```python
from build123d import *

# Parameters (mm, degrees)
EXTRUDE_1_DEPTH          = 30
CUT_EXTRUDE_1_DEPTH      = 301
CUT_EXTRUDE_2_DEPTH      = 12
CUT_EXTRUDE_2_DEPTH_BACK = 12


with BuildPart() as part:
    # Эскиз1 → Бобышка-Вытянуть1 (new body)
    with BuildSketch(Plane.XY):
        Polygon((0, 0), (300, 0), (300, 25), (0, 50), align=None)
    extrude(amount=EXTRUDE_1_DEPTH)

    # Эскиз2 → Вырез-Вытянуть1 (cut, through all)
    with BuildSketch(Plane(origin=(300, 0, 0), x_dir=(0, 0, -1), z_dir=(1, 0, 0))):
        Polygon((-18.429564861, 0), (-18.429564861, 1.797684404), (-28.323382455, 1.797684404), (-28.323382455, 11.297500412), (-1.676617545, 11.297500412), (-1.676617545, 1.797684404), (-11.570435139, 1.797684404), (-11.570435139, 0), align=None)
    extrude(amount=-CUT_EXTRUDE_1_DEPTH, mode=Mode.SUBTRACT)

    # Эскиз3 → Вырез-Вытянуть2 (cut, two sides)
    with BuildSketch(Plane(origin=(0, 0, 15), x_dir=(-1, 0, 0), z_dir=(0, 0, -1))) as cut_extrude_2_sk:
        Polygon((-300, 7.808397482), (0, 7.808397482), (0, 47.550024082), (-300, 23.437127044), align=None)
    extrude(amount=CUT_EXTRUDE_2_DEPTH, mode=Mode.SUBTRACT)
    extrude(cut_extrude_2_sk.sketch, amount=-CUT_EXTRUDE_2_DEPTH_BACK, mode=Mode.SUBTRACT)


solid = part.part
```
Geometry: final body of the model. Coordinates: model frame, mm. A direction names the side the tool comes from. Give positions to 0.01 mm unless a question says otherwise; leave off trailing zeros. Loops run counter-clockwise (first coordinate to the right, second up) from the corner with the lowest first, then second, coordinate; pieces in that order, holes last. Notation, with made-up numbers: (-28.75, 77) -> (-0.75, 77) arc R29 cw to (-0.75, 113) -> close; hole circle Ø10 at (-17, -33.5). An arc over 180 degrees is marked (long way). Return JSON: item names as keys, results as strings.
Item 1: Section C-C, the plane x = 268.5. Output: boundary loops of the cut face in (y, z) (1 decimal), plus the area to 3 significant figures.
Filled in:
{"outline": "(0, 0) -> (27.6, 0) -> (27.6, 30) -> (0, 30) -> (0, 18.4) -> (1.8, 18.4) -> (1.8, 28.3) -> (11.3, 28.3) -> (11.3, 27) -> (26, 27) -> (26, 3) -> (11.3, 3) -> (11.3, 1.7) -> (1.8, 1.7) -> (1.8, 11.6) -> (0, 11.6) -> close", "area": "211 mm^2"}
Item 2: Mould query, pull axis Y, two halves, no side actions, for faces 4 (the flat face through (300, 24, 14)), 5 (the flat face through (119, 26, 3)), 6 (the flat face through (148, 0, 24)). Classes: released by +Y, released by -Y, zero draft, split by the parting line, or undercut.
Filled in:
{"face 4": "zero draft", "face 5": "undercut", "face 6": "released by -Y"}
Item 3: Access query for faces 1 (the flat face through (152.1, 37.325, 14.79)), 2 (the flat face through (152, 1.798, 7)), 3 (the flat face through (147.9, 35.662, 14.832)). Directions: +Z, -Z, +X, -X, +Y, -Y. A direction counts if a zero-diameter tool reaches every point of the face in a straight line with its end or side. Return the directions, or none.
Filled in:
{"face 1": "+Z, -Z, +X, +Y", "face 2": "+X, -X", "face 3": "-X"}
Item 4: Section D-D, the plane y = 41.5. Output: boundary loops of the cut face in (x, z).
Filled in:
{"outline": "(0, 0) -> (102, 0) -> (102, 30) -> (0, 30) -> (0, 27) -> (75.27, 27) -> (75.27, 3) -> (0, 3) -> close"}
Item 5: Line query: line 1 (Z direction, x = 130, y = 24.5); line 2 (Z direction, x = 51.5, y = 7); line 3 (Y direction, x = 265, z = 25.5). Output: solid intervals per line, ascending.
Filled in:
{"line 1": "0 to 3, 27 to 30", "line 2": "0 to 1.68, 28.32 to 30", "line 3": "0 to 1.8, 26.25 to 27.92"}
Item 6: Section B-B, the plane y = 14.5. Output: boundary loops of the cut face in (x, z).
Filled in:
{"outline": "(0, 0) -> (300, 0) -> (300, 3) -> (0, 3) -> close; (0, 27) -> (300, 27) -> (300, 30) -> (0, 30) -> close"}
Item 7: Section A-A, the plane z = 23.5. Output: boundary loops of the cut face in (x, y), plus the area to 3 significant figures.
Filled in:
{"outline": "(0, 0) -> (300, 0) -> (300, 1.8) -> (0, 1.8) -> close; (0, 47.55) -> (300, 23.44) -> (300, 25) -> (0, 50) -> close", "area": "1,140 mm^2"}
Item 8: Pin query (flat end, axial travel): P1, Ø1, axis at x = 130.5, z = 12, coming from the +Y side; P2, Ø1.5, axis at x = 152, z = 21, coming from the +Y side; P3, Ø8, axis at y = 15.5, z = 15.5, coming from the -X side; P4, Ø3, axis at x = 144.5, z = 4.5, coming from the +Y side. Return the tip coordinate at first contact, or that it passes through.
Filled in:
{"P1": "y = 39.17", "P2": "y = 37.4", "P3": "through", "P4": "y = 38.08"}
